Verification items for the finished model (mm, model axes). A direction names the side the tool comes from. Coordinates: 2 decimals unless noted, no trailing zeros. Order: outer loops, then holes, each group sorted by start corner. A loop starts at its lowest first (then second) coordinate and runs counter-clockwise, first axis right, second up. Notation, with made-up numbers: (-33.75, -39.5) - (20.25, -39.5) arc R6 cw to (20.25, -32.5) - close; hole circle Ø10 at (89, 45.5). An arc over 180 degrees is marked (long way). Answer as CSV lines item,"result". Start each with the question number.
1. Set-up check for faces 4 (the flat face through (18, 1.587, 18)), 5 (the cylindrical face through (25.593, 2.601, 31.287)), 6 (the flat face through (12.076, 2.601, 17.748)): record each of +Z, -Z, +X, -X, +Y, -Y from which the full face is reachable in a straight line by a thin tool's end or side.
2. Section check D-D (x = 21.5). Record the cut outline in (y, z).
3. Material ranges on L1, parallel to Z at x = 0, y = 1.1; L2, parallel to X at y = 1.95, z = 3; L3, parallel to X at y = 0.2, z = 18, recorded low to high. Write a range as [from, to].
4. Mould release check, pull along Z, two halves, no side actions. Record for faces 1 (the flat face through (-10, 1, 3)), 2 (the flat face through (0, 1, 6)), 3 (the cylindrical face through (-17.194, 2.601, 4.787)): pulls with the +Z half, pulls with the -Z half, needs draft (parallel to the pull), parting line crosses it, or undercut.
5. Section check A-A (z = 2.5). Record the cut outline in (x, y), and give its area (3 significant figures).
6. Section check C-C (z = 31.25). Record the cut outline in (x, y).
7. Section check B-B (x = 0). Record the cut outline in (y, z), and give its area (3 significant figures).
8. Go/stop test with flat-tipped pins: pin 1 (1 mm diameter, centred on x = -20.5, y = 2.5, fed in from -Z); pin 2 (11 mm diameter, centred on x = -25, z = 23.5, fed in from -Y); pin 3 (10 mm diameter, centred on x = -3.5, z = 16.5, fed in from +Y); pin 4 (0.6 mm diameter, centred on y = 1, z = 3, fed in from -X). Record where each tip stops, or that it passes through.
Autodesk Inventor part; units mm, degrees
ref_plane "YZ Plane" through (0, 0, 0) normal (1, 0, 0) x (0, 1, 0)
ref_plane "XZ Plane" through (0, 0, 0) normal (0, 1, 0) x (-1, 0, 0)
ref_plane "XY Plane" through (0, 0, 0) normal (0, 0, 1) x (1, 0, 0)
sketch "草圖1" plane through (0, 0, 0) normal (0, 0, 1) x (1, 0, 0)
  line L0 (-22.5, 3.5874) -> (-14.0953, 3.5874)
  line L1 (-14.0953, 3.5874) -> (-10, 1.5874)
  line L2 (-10, 1.5874) -> (0, 1.5874)
  line L3 (0.691, -0.4126) -> (-10.4623, -0.4126)
  line L4 (-10.4623, -0.4126) -> (-14.5576, 1.5874)
  line L5 (-14.5576, 1.5874) -> (-22.5, 1.5874)
  line L6 (-22.5, 1.5874) -> (-22.5, 3.5874)
  line L7 (0, 2.1547) -> (0, -6.606) construction
  line L8 (22.5, 3.5874) -> (14.0953, 3.5874)
  line L9 (14.0953, 3.5874) -> (10, 1.5874)
  line L10 (10, 1.5874) -> (0, 1.5874)
  line L11 (0.691, -0.4126) -> (10.4623, -0.4126)
  line L12 (10.4623, -0.4126) -> (14.5576, 1.5874)
  line L13 (14.5576, 1.5874) -> (22.5, 1.5874)
  line L14 (22.5, 1.5874) -> (22.5, 3.5874)
  line L15 (-22.25, -3.3995) -> (-22.25, 2.4631)
  line L16 (22.25, -3.2727) -> (22.25, 2.4631)
  line L17 (10, -4.4814) -> (10, 6.978)
  point P0 (0, 0)
  point P1 (-22.25, 1.5321)
  point P2 (22.25, 1.5874)
  point P3 (22.25, 1.5321)
  dimension "d1" = 2
  dimension "d5" = 44.5
  dimension "d9" = 45
  dimension "d32" = 10
  dimension "d36" = 2
  dimension "d46" = 2
extrude "擠出1" add sketch "草圖1" along normal blind 36
sketch "草圖2" plane through (-22.5, 3.5874, 0) normal (0, 1, 0) x (1, 0, 0)
  point P0 (22.5, 0)
sketch "草圖3" plane through (-22.5, 3.5874, 0) normal (0, 1, 0) x (1, 0, 0)
  line L0 (0, 0) -> (0, -36)
  line L1 (0, 0) -> (0, -10.4873)
  line L2 (0, 0) -> (-6, 0)
  line L3 (-6, 0) -> (-6, -8.018)
  line L4 (-6, -36) -> (0, -36)
  line L5 (-6, -27.982) -> (-6, -36)
  line L6 (22.5, -5.8594) -> (22.5, -37.147)
  arc A0 (0, -10.4873) -> (-6, -8.018) centre (-6.6, -18) ccw
  arc A1 (-6, -27.982) -> (0, -10.4873) centre (-6.6, -18) ccw
  line L7 (0, -25.5127) -> (0, -36)
  line L8 (45, 0) -> (45, -36)
  line L9 (45, 0) -> (45, -10.4873)
  line L10 (45, 0) -> (51, 0)
  line L11 (51, 0) -> (51, -8.018)
  line L12 (51, -36) -> (45, -36)
  line L13 (51, -27.982) -> (51, -36)
  arc A2 (51, -8.018) -> (45, -10.4873) centre (51.6, -18) ccw
  arc A3 (45, -10.4873) -> (51, -27.982) centre (51.6, -18) ccw
  line L14 (45, -25.5127) -> (45, -36)
  line L15 (-7.7403, -18) -> (53.0258, -18)
  point P0 (22.5, 0)
  point P1 (45, -25.5127)
  point P2 (-6, -4.009)
  dimension "d13" = 6.6
  dimension "d18" = 45
  dimension "d19" = 6
  dimension "d20" = 6
  dimension "d37" = 10
  dimension "d47" = 36
extrude "擠出2" add sketch "草圖3" against normal blind 2 contours L8 L10 L11 A2 | A3 L13 L12 L8 | L0 L4 L5 A1 | L0 A0 L3 L2
extrude "擠出3" cut sketch "草圖3" against normal blind 2.5 contours A3 L8 L15 | L15 L8 A3 | A1 L15 L0 | L15 A1 L0
sketch "草圖4" plane through (-14.0953, 3.5874, 36) normal (0, 1, 0) x (1, 0, 0)
  line L0 (-14.4047, 36) -> (-0.4623, 36)
  line L1 (-8.1547, 36) -> (-8.1547, -2.5095)
  line L2 (-14.4047, 36) -> (-14.4047, 27.982)
  line L3 (28.1906, 0) -> (42.5953, 0)
  line L4 (-9.798, 31.25) -> (-4.798, 31.25) construction
  line L5 (-9.798, 29.55) -> (-4.798, 29.55)
  line L6 (-4.798, 32.95) -> (-9.798, 32.95)
  arc A0 (-9.798, 32.95) -> (-9.798, 29.55) centre (-9.798, 31.25) ccw
  arc A1 (-4.798, 29.55) -> (-4.798, 32.95) centre (-4.798, 31.25) ccw
  line L7 (-25.514, 18) -> (67.1526, 18)
  line L8 (14.0953, -5.2274) -> (14.0953, 45.8177)
  circle A2 centre (14.0953, 18) radius 6.5
  line L9 (-9.798, 4.75) -> (-4.798, 4.75) construction
  line L10 (-9.798, 6.45) -> (-4.798, 6.45)
  line L11 (-4.798, 3.05) -> (-9.798, 3.05)
  arc A3 (-9.798, 6.45) -> (-9.798, 3.05) centre (-9.798, 4.75) ccw
  arc A4 (-4.798, 3.05) -> (-4.798, 6.45) centre (-4.798, 4.75) ccw
  line L12 (37.9886, 31.25) -> (32.9886, 31.25) construction
  line L13 (37.9886, 29.55) -> (32.9886, 29.55)
  line L14 (32.9886, 32.95) -> (37.9886, 32.95)
  arc A5 (37.9886, 29.55) -> (37.9886, 32.95) centre (37.9886, 31.25) ccw
  arc A6 (32.9886, 32.95) -> (32.9886, 29.55) centre (32.9886, 31.25) ccw
  arc A7 (32.9886, 6.45) -> (32.9886, 3.05) centre (32.9886, 4.75) ccw
  line L15 (37.9886, 6.45) -> (32.9886, 6.45)
  line L16 (37.9886, 4.75) -> (32.9886, 4.75) construction
  arc A8 (37.9886, 3.05) -> (37.9886, 6.45) centre (37.9886, 4.75) ccw
  line L17 (32.9886, 3.05) -> (37.9886, 3.05)
  point P0 (14.0953, 36)
  point P1 (-7.298, 31.25)
  point P2 (-7.298, 4.75)
  point P3 (35.4886, 31.25)
  point P4 (35.4886, 4.75)
  dimension "d21" = 6.25
  dimension "d33" = 3.4
  dimension "d48" = 36
  dimension "d49" = 13
  dimension "d52" = 26.5
  dimension "d53" = 9.2134
  dimension "d54" = 5
extrude "擠出4" cut sketch "草圖4" against normal up to surface (4 mm away)
sketch "草圖5" plane through (-10, 1.5874, 0) normal (0, 1, 0) x (1, 0, 0)
  line L0 (-0.4623, 0) -> (20.4623, 0)
  line L1 (0, 0) -> (20, 0)
  line L2 (20, 0) -> (20, -6)
  line L3 (20, -6) -> (0, -6)
  line L4 (0, -6) -> (0, 0)
  line L5 (10, -2.0229) -> (10, 3.2313)
  point P0 (10, 0)
  point P1 (20, 0)
  point P2 (20, 0)
  point P3 (10, 0)
  dimension "d38" = 6
  dimension "d42" = 20
extrude "擠出5" cut sketch "草圖5" against normal up to surface (2 mm away)
fillet "圓角2" radius 1 4 edges at (-10, 0.5874, 0) (10, 0.5874, 0) (-10, 0.5874, 6) (10, 0.5874, 6)
properties part number "連接件"
Evaluation:
1,face 4,"+Z, -Z, +X, -Y"
1,face 5,"+Y, -Y"
1,face 6,"+Z, -Z, +Y"
2,outline,"(1.59, 0) - (3.59, 0) - (3.59, 3.05) - (1.59, 3.05) - close; (1.59, 6.45) - (3.59, 6.45) - (3.59, 11.5) - (1.59, 11.5) - close; (1.59, 24.5) - (3.59, 24.5) - (3.59, 29.55) - (1.59, 29.55) - close; (1.59, 32.95) - (3.59, 32.95) - (3.59, 36) - (1.59, 36) - close"
3,L1,"z = [6, 11.5], [24.5, 36]"
3,L2,"x = [-28.5, -10.74], [10.74, 28.5]"
3,L3,"x = [-11.72, -6.5], [6.5, 11.72]"
4,face 1,"needs draft"
4,face 2,"pulls with the -Z half"
4,face 3,"undercut"
5,outline,"(-28.5, 1.59) - (-14.56, 1.59) - (-10.46, -0.41) - (-10, -0.41) - (-10, 1.59) - (-14.1, 3.59) - (-28.5, 3.59) - close; (10, -0.41) - (10.46, -0.41) - (14.56, 1.59) - (28.5, 1.59) - (28.5, 3.59) - (14.1, 3.59) - (10, 1.59) - close"
5,area,"75.8 mm²"
6,outline,"(-28.5, 1.59) - (-25.59, 1.59) - (-25.59, 3.59) - (-28.5, 3.59) - close; (-17.19, 1.59) - (-14.56, 1.59) - (-10.46, -0.41) - (10.46, -0.41) - (14.56, 1.59) - (17.19, 1.59) - (17.19, 3.59) - (14.1, 3.59) - (10, 1.59) - (-10, 1.59) - (-14.1, 3.59) - (-17.19, 3.59) - close; (25.59, 1.59) - (28.5, 1.59) - (28.5, 3.59) - (25.59, 3.59) - close"
7,outline,"(-0.41, 6) - (1.59, 6) - (1.59, 11.5) - (-0.41, 11.5) - close; (-0.41, 24.5) - (1.59, 24.5) - (1.59, 36) - (-0.41, 36) - close"
7,area,"34.0 mm²"
8,pin 1,"stops at z = 0"
8,pin 2,"stops at y = 1.59"
8,pin 3,"stops at y = 1.59"
8,pin 4,"stops at x = -13.97"
